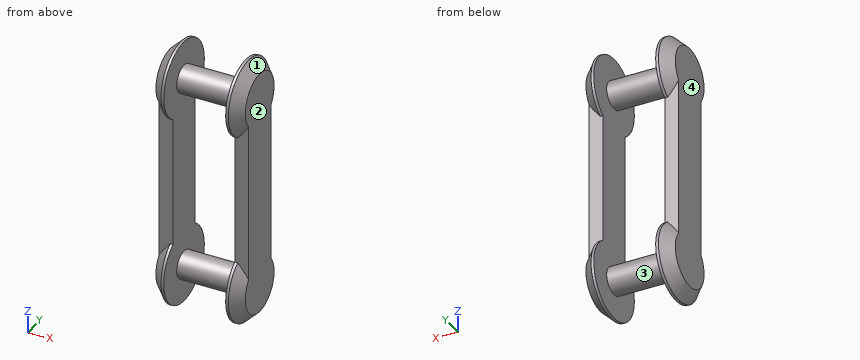
```python
from build123d import *

# Parameters (mm, degrees)
F0_R     = 6.35
F1_DEPTH = 14.2875
F3_DEPTH = 6.35
F4_SIZE  = 5.08
F5_R     = 6.35
F6_DEPTH = 28.575


with BuildPart() as f1:
    # F0 (on Right) → F1 (new body, symmetric)
    with BuildSketch(Plane.YZ):
        Circle(F0_R)
    extrude(amount=F1_DEPTH, both=True)

    # F2 (on face) → F3 (join)
    with BuildSketch(Plane.YZ.offset(14.2875)):
        with BuildLine():
            Line((9.525, 88.9), (9.525, 74.263973174))
            ThreePointArc((9.525, 74.263973174), (15.3503944371, 80.5750797676), (17.4625, 88.9))
            ThreePointArc((17.4625, 88.9), (-8.3249202324, 104.2503944371), (-9.525, 74.263973174))
            Line((-9.525, 74.263973174), (-9.525, 88.9))
            Line((-9.525, 88.9), (9.525, 88.9))
        make_face()
        with BuildLine():
            ThreePointArc((-9.525, 74.263973174), (0, 71.4375), (9.525, 74.263973174))
            Line((9.525, 74.263973174), (9.525, 88.9))
            Line((9.525, 88.9), (-9.525, 88.9))
            Line((-9.525, 88.9), (-9.525, 74.263973174))
        make_face()
        with BuildLine():
            ThreePointArc((-9.525, 14.636026826), (0, 17.4625), (9.525, 14.636026826))
            Line((9.525, 14.636026826), (9.525, 74.263973174))
            ThreePointArc((9.525, 74.263973174), (0, 71.4375), (-9.525, 74.263973174))
            Line((-9.525, 74.263973174), (-9.525, 14.636026826))
        make_face()
        with BuildLine():
            Line((9.525, 0), (9.525, 14.636026826))
            ThreePointArc((9.525, 14.636026826), (0, 17.4625), (-9.525, 14.636026826))
            Line((-9.525, 14.636026826), (-9.525, 0))
            Line((-9.525, 0), (-6.35, 0))
            ThreePointArc((-6.35, 0), (0, 6.35), (6.35, 0))
            Line((6.35, 0), (9.525, 0))
        make_face()
        with BuildLine():
            ThreePointArc((-6.35, 0), (0, -6.35), (6.35, 0))
            Line((6.35, 0), (-6.35, 0))
        make_face()
        with BuildLine():
            ThreePointArc((-9.525, 14.636026826), (-8.3249202324, -15.3503944371), (17.4625, 0))
            ThreePointArc((17.4625, 0), (15.3503944371, 8.3249202324), (9.525, 14.636026826))
            Line((9.525, 14.636026826), (9.525, 0))
            Line((9.525, 0), (6.35, 0))
            ThreePointArc((6.35, 0), (0, -6.35), (-6.35, 0))
            Line((-6.35, 0), (-9.525, 0))
            Line((-9.525, 0), (-9.525, 14.636026826))
        make_face()
        with BuildLine():
            Line((-6.35, 0), (6.35, 0))
            ThreePointArc((6.35, 0), (0, 6.35), (-6.35, 0))
        make_face()
    extrude(amount=F3_DEPTH)

    # F4
    f4_edges = [f1.edges().sort_by_distance(p)[0] for p in [
        (20.6375, 0, 106.3625),
        (20.6375, 0, -17.4625),
    ]]
    chamfer(f4_edges, length=F4_SIZE)

    # F5 (on face) → F6 (join)
    with BuildSketch(Plane(origin=(14.2875, 0, 0), x_dir=(0, -1, 0), z_dir=(-1, 0, 0))):
        with Locations((0, 88.9)):
            Circle(F5_R)
    extrude(amount=F6_DEPTH)

    # F7: F1 across plane


with BuildPart() as f1_1:
    add(f1.part)
    add(f1.part.mirror(Plane.YZ))


solid = f1_1.part
```
Read the model definition and answer for the solid it produces. Units are mm, in the model's axes. Face numbers are marked on the shaded views. A direction names the side the tool comes from. Give positions to 0.01 mm unless a question says otherwise; leave off trailing zeros. Write each loop counter-clockwise with the first axis right and the second up, starting at its lowest first coordinate (ties: lowest second). Pieces come first, ordered by that corner, then holes. Notation, with made-up numbers: M 83,52 L 136,52 A13 ccw 136,58 Z; hole C -37.5,42 d1. An arc over 180 degrees is marked long. Put each result on its own line as item: value. Start each with the question number.
1. The part is cut by section B-B, the plane z = 58. Give the vertices of the cut face in (x, y) (1 decimal), and give its area (3 significant figures).
2. Consider line 1 along X through (y, z) = (-6, 23); line 2 along Z through (x, y) = (-15, 11); line 3 along X through (y, z) = (9.5, -11.5). Determine where each line is inside the solid, lowest interval first.
3. Each of these flat-tipped pins is pushed along its axis until it touches: pin 1 Ø1.9 at (x, z) = (-18.5, 42.5) entering from -Y (3 decimals); pin 2 Ø2 at (x, y) = (12.5, 13) entering from +Z; pin 3 Ø7 at (x, z) = (-16.5, 58.5) entering from +Y (3 decimals); pin 4 Ø4 at (x, y) = (-10, 3) entering from +Z. Where does it stop, or does it pass through?
4. For a pull along Z with two mould halves and no side action, classify the marked faces 1 and 2 as released by +Z, released by -Z, zero draft, split by the parting line, or undercut.
5. Which of the six approach directions +Z, -Z, +X, -X, +Y, -Y give full straight-line access (tool end or side, diameter ignored) to the marked faces 3 and 4?
6. The part is cut by section A-A, the plane y = 0. Give the vertices of the cut face in (x, z), and give its area (3 significant figures).
7. The part is cut by section D-D, the plane z = 0. Give the vertices of the cut face in (x, y).
8. The part is cut by section C-C, the plane x = -13. Give the vertices of the cut face in (y, z).
Final values:
1. outline: M -20.6,-9.5 L -14.3,-9.5 L -14.3,9.5 L -20.6,9.5 Z; M 14.3,-9.5 L 20.6,-9.5 L 20.6,9.5 L 14.3,9.5 Z
1. area: 242 mm²
2. line 1: x = -20.64 to -14.29, 14.29 to 20.64
2. line 2: z = -13.56 to 13.56, 75.34 to 102.46
2. line 3: x = -18.1 to -14.29, 14.29 to 18.1
3. pin 1: stops at y = -9.525
3. pin 2: passes through
3. pin 3: stops at y = 9.525
3. pin 4: stops at z = 95.17
4. face 1: undercut
4. face 2: zero draft
5. face 3: none
5. face 4: +Z, -Z, -X, +Y, -Y
6. outline: M -20.64,-12.38 L -15.56,-17.46 L -14.29,-17.46 L -14.29,-6.35 L 14.29,-6.35 L 14.29,-17.46 L 15.56,-17.46 L 20.64,-12.38 L 20.64,101.28 L 15.56,106.36 L 14.29,106.36 L 14.29,95.25 L -14.29,95.25 L -14.29,106.36 L -15.56,106.36 L -20.64,101.28 Z; hole M -14.29,6.35 L 14.29,6.35 L 14.29,82.55 L -14.29,82.55 Z
6. area: 2,250 mm²
7. outline: M -20.64,-12.38 L -15.56,-17.46 L -14.29,-17.46 L -14.29,-6.35 L 14.29,-6.35 L 14.29,-17.46 L 15.56,-17.46 L 20.64,-12.38 L 20.64,12.38 L 15.56,17.46 L 14.29,17.46 L 14.29,6.35 L -14.29,6.35 L -14.29,17.46 L -15.56,17.46 L -20.64,12.38 Z
8. outline: C 0,0 d12.7; C 0,88.9 d12.7
